Part model, mm, in its own coordinate system. A direction names the side the tool comes from. Coordinates: 2 decimals unless noted, no trailing zeros. Order: outer loops, then holes, each group sorted by start corner. A loop starts at its lowest first (then second) coordinate and runs counter-clockwise, first axis right, second up.
```python
from build123d import *

# Parameters (mm, degrees)
F0_R     = 1.5
F0_W     = 3.8139913231
F0_H     = 2
F1_DEPTH = 3
F2_DEPTH = 35
F3_DEPTH = 25


with BuildPart() as f1:
    # F0 (on Front) → F1 (new body)
    with BuildSketch(Plane.XZ):
        Polygon((7, -9.8663857207), (7, 0), (0, -9), (0, -15), (24, -15), (24, -9), (17, 0), (16.9568490237, -9.8663857207), align=None)
        with Locations((4, -12)):
            Circle(F0_R, mode=Mode.SUBTRACT)
        with Locations((20, -12)):
            Circle(F0_R, mode=Mode.SUBTRACT)
        Polygon((10.1258195937, 0), (7, 0), (7, -9.8663857207), (16.9568490237, -9.8663857207), (17, 0), (13.9398109168, 0), (13.9398109168, -2), (15, -2), (15, -8), (9, -8), (9, -2), (10.1258195937, -2), align=None)
        with Locations((12.0328152552, -1)):
            Rectangle(F0_W, F0_H)
        Polygon((13.9398109168, -2), (10.1258195937, -2), (9, -2), (9, -8), (15, -8), (15, -2), align=None)
    extrude(amount=-F1_DEPTH)

    # F0 (on Front) → F2 (join)
    with BuildSketch(Plane.XZ):
        Polygon((10.1258195937, 0), (7, 0), (7, -9.8663857207), (16.9568490237, -9.8663857207), (17, 0), (13.9398109168, 0), (13.9398109168, -2), (15, -2), (15, -8), (9, -8), (9, -2), (10.1258195937, -2), align=None)
        Polygon((13.9398109168, -2), (10.1258195937, -2), (9, -2), (9, -8), (15, -8), (15, -2), align=None)
        with Locations((12.0328152552, -1)):
            Rectangle(F0_W, F0_H)
    extrude(amount=-F2_DEPTH)

    # F0 (on Front) → F3 (cut)
    with BuildSketch(Plane.XZ):
        with Locations((12.0328152552, -1)):
            Rectangle(F0_W, F0_H)
        Polygon((13.9398109168, -2), (10.1258195937, -2), (9, -2), (9, -8), (15, -8), (15, -2), align=None)
    extrude(amount=-F3_DEPTH, mode=Mode.SUBTRACT)


solid = f1.part
```
(1) Slice it at A-A, the plane x = 3.75. Give the cut face in (y, z), then the cut area to 3 significant figures.
(2) Slice it at D-D, the plane x = 15.75. Give the cut face in (y, z), then the cut area to 3 significant figures.
(3) Probe line 1 (Z direction, x = 9.75, y = 19.5); line 2 (Z direction, x = 8.5, y = 17.5); line 3 (Y direction, x = 12, z = -12.75). List the from-to ranges inside material, lowest first.
(4) Slice it at B-B, the plane z = -12. Give the cut face in (x, y), then the cut area to 3 significant figures.
(5) Tool access for faces 4 (the face through (0, 1, -12)), 5 (the face through (12, 19, -9.866)), 6 (the face through (9, 12, -5)): list every direction of +Z, -Z, +X, -X, +Y, -Y with a clear straight run to the whole face (end or side of a thin tool).
(6) Pull direction X, two halves, no side cores. Call faces 1 (the face through (7, 19, -5)), 2 (the face through (12, 1, -15)), 3 (the face through (13.94, 12, -1)): +X half, -X half, draft (parallel to the pull), parting line (faces both ways), or undercut.
(7) Drop flat-ended pins along their axis: pin 1 (0.5 mm diameter, centred on x = 14.5, y = 17.5, fed in from -Z); pin 2 (5 mm diameter, centred on y = 26, z = -3.5, fed in from -X); pin 3 (1.8 mm diameter, centred on y = 11.5, z = -6, fed in from +X); pin 4 (2.5 mm diameter, centred on x = 4, z = -12, fed in from -Y). Give the stop position or say it passes through.
(8) Slice it at C-C, the plane y = 7.5. Give the cut face in (x, z), then the cut area to 3 significant figures.
Here are the results:
1. outline: (0, -15) - (3, -15) - (3, -13.48) - (0, -13.48) - close; (0, -10.52) - (3, -10.52) - (3, -4.18) - (0, -4.18) - close
1. area: 23.6 mm2
2. outline: (0, -15) - (3, -15) - (3, -9.87) - (35, -9.87) - (35, 0) - (0, 0) - close
2. area: 361 mm2
3. line 1: z = -9.87 to -8, -2 to 0
3. line 2: z = -9.87 to 0
3. line 3: y = 0 to 3
4. outline: (0, 0) - (2.5, 0) - (2.5, 3) - (0, 3) - close; (5.5, 0) - (18.5, 0) - (18.5, 3) - (5.5, 3) - close; (21.5, 0) - (24, 0) - (24, 3) - (21.5, 3) - close
4. area: 54.0 mm2
5. face 4: +Z, -Z, -X, +Y, -Y
5. face 5: -Z, +X, -X, +Y
5. face 6: -Y
6. face 1: -X half
6. face 2: draft
6. face 3: undercut
7. pin 1: stops at z = -9.87
7. pin 2: stops at x = 7
7. pin 3: stops at x = 16.98
7. pin 4: passes through
8. outline: (7, -9.87) - (16.96, -9.87) - (17, 0) - (13.94, 0) - (13.94, -2) - (15, -2) - (15, -8) - (9, -8) - (9, -2) - (10.13, -2) - (10.13, 0) - (7, 0) - close
8. area: 54.8 mm2
